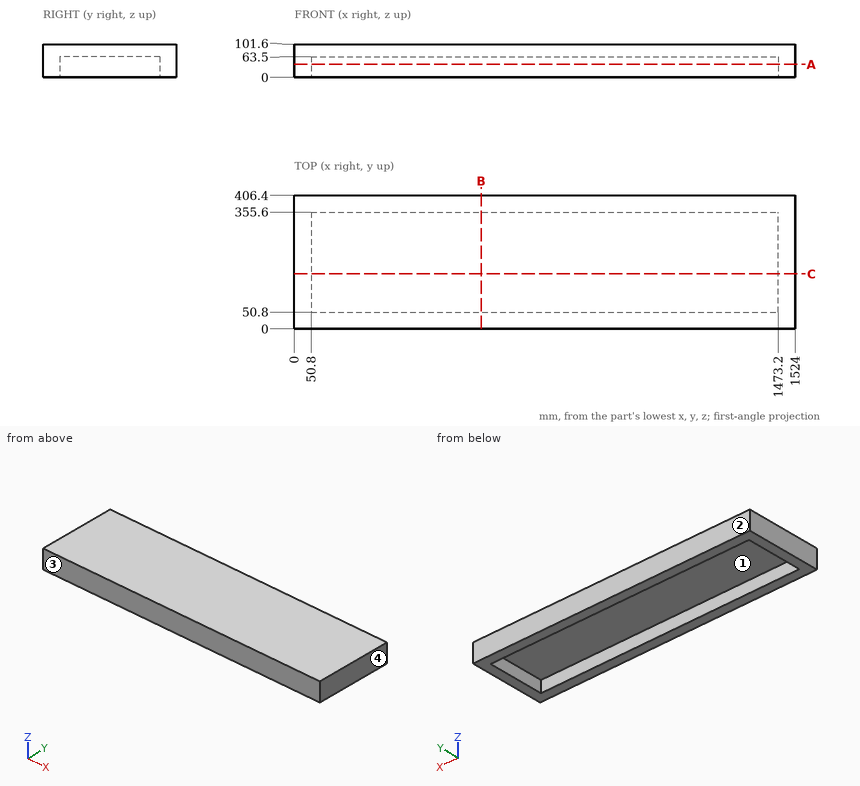
Geometry check sheet. Reference: drawing and pictorial views, mm from the part's lowest x, y, z. Give positions to 0.01 mm unless a question says otherwise; leave off trailing zeros. Write each loop counter-clockwise with the first axis right and the second up, starting at its lowest first coordinate (ties: lowest second). Pieces come first, ordered by that corner, then holes. Notation, with made-up numbers: M 55,-13 L 99,-13 A9 cw 99,-9 Z; hole C -8,-35.75 d3. An arc over 180 degrees is marked long. Put each result on its own line as item: value. Start each with the question number.
1. Go/stop test with a flat-tipped pin: pin 1 Ø5 at (x, y) = (501.5, 202.5) entering from -Z. Record where the tip stops, or that it passes through.
2. Section check A-A (z = 39.5). Record the cut outline in (x, y), and give its area (3 significant figures).
3. Scan lines: line 1 along Y through (x, z) = (1124.5, 55); line 2 along X through (y, z) = (191, 16); line 3 along Z through (x, y) = (941.5, 215). Record each from-to range of solid material in increasing order. Write a range as [from, to].
4. Section check B-B (x = 568.5). Record the cut outline in (y, z), and give its area (3 significant figures).
5. Section check C-C (y = 167.5). Record the cut outline in (x, z).
6. Draft check along Y on the marked faces 1, 2, 3 and 4. Enter one of: +Y half, -Y half, draft (parallel to the pull), parting line (faces both ways), or undercut.
Answer list:
1. pin 1: z = 63.5
2. outline: M 0,0 L 1524,0 L 1524,406.4 L 0,406.4 Z; hole M 50.8,50.8 L 1473.2,50.8 L 1473.2,355.6 L 50.8,355.6 Z
2. area: 186,000 mm2
3. line 1: [0, 50.8], [355.6, 406.4]
3. line 2: [0, 50.8], [1473.2, 1524]
3. line 3: [63.5, 101.6]
4. outline: M 0,0 L 50.8,0 L 50.8,63.5 L 355.6,63.5 L 355.6,0 L 406.4,0 L 406.4,101.6 L 0,101.6 Z
4. area: 21,900 mm2
5. outline: M 0,0 L 50.8,0 L 50.8,63.5 L 1473.2,63.5 L 1473.2,0 L 1524,0 L 1524,101.6 L 0,101.6 Z
6. face 1: undercut
6. face 2: +Y half
6. face 3: -Y half
6. face 4: draft
